Autodesk Inventor part; units mm, degrees
ref_plane "YZ Plane" through (0, 0, 0) normal (1, 0, 0) x (0, 1, 0)
ref_plane "XZ Plane" through (0, 0, 0) normal (0, 1, 0) x (-1, 0, 0)
ref_plane "XY Plane" through (0, 0, 0) normal (0, 0, 1) x (1, 0, 0)
sketch "Sketch1" plane through (0, 0, 0) normal (0, 1, 0) x (-1, 0, 0)
  line L0 (46.6228, 34.6302) -> (-74.0272, 34.6302)
  line L1 (-74.0272, 34.6302) -> (-74.0272, -28.8698)
  line L2 (-74.0272, -28.8698) -> (46.6228, -28.8698)
  line L3 (46.6228, -28.8698) -> (46.6228, 34.6302)
  point P0 (0, 0)
  dimension "d0" = 120.65
  dimension "d1" = 63.5
extrude "Extrusion1" add sketch "Sketch1" along normal blind 12.7
sketch "Sketch2" plane through (0, 12.7, 0) normal (0, 1, 0) x (1, 0, 0)
  line L0 (-46.6228, -34.6302) -> (74.0272, -34.6302)
  line L1 (-46.6228, 28.8698) -> (-46.6228, -34.6302)
  point P0 (0, 0)
  point P1 (4.1772, -18.7552)
  point P2 (54.9772, -18.7552)
  dimension "d4" = 0
  dimension "d5" = 15.875
  dimension "d6" = 50.8
  dimension "d7" = 50.8
hole "Hole1" at (4.1772, 12.7, 18.7552) at (54.9772, 12.7, 18.7552) direction (0, -1, 0) diameter 4.826 depth 25.4 tip angle 118 countersink diameter 9.525 countersink angle 82
sketch "Sketch3" plane through (0, 0, 0) normal (0, -1, 0) x (1, 0, 0)
  line L0 (-16.8428, 29.5502) -> (-28.8428, 29.5502)
  line L1 (-28.8428, 29.5502) -> (-28.8428, 23.5502)
  line L2 (-28.8428, 23.5502) -> (-16.8428, 23.5502)
  line L3 (-16.8428, 23.5502) -> (-16.8428, 29.5502)
  line L4 (-46.6228, 34.6302) -> (74.0272, 34.6302)
  line L5 (-46.6228, -28.8698) -> (-46.6228, 34.6302)
  point P0 (0, 0)
  dimension "d15" = 6
  dimension "d16" = 12
  dimension "d17" = 5.08
  dimension "d18" = 17.78
extrude "Extrusion2" cut sketch "Sketch3" against normal blind 1.27
sketch "Sketch4" plane through (0, 0, 0) normal (0, -1, 0) x (1, 0, 0)
  line L0 (74.0272, -28.8698) -> (-46.6228, -28.8698)
  line L1 (-28.8428, 23.5502) -> (-28.8428, 29.5502)
  line L2 (-46.6228, -28.8698) -> (-46.6228, 34.6302)
  point P0 (0, 0)
  point P1 (-32.8428, -16.6898)
  point P2 (-32.8428, -23.7898)
  point P3 (-11.9428, -23.7898)
  point P4 (-11.9428, -16.6898)
  dimension "d21" = 0
  dimension "d22" = 0
  dimension "d23" = 0
  dimension "d24" = 0
  dimension "d25" = 5.08
  dimension "d26" = 7.1
  dimension "d27" = 20.9
  dimension "d35" = 4
  dimension "d92" = 13.78
hole "Hole2" at (-32.8428, 0, -16.6898) at (-32.8428, 0, -23.7898) at (-11.9428, 0, -23.7898) at (-11.9428, 0, -16.6898) direction (0, 1, 0) diameter 2.8 depth 25.4 tip angle 118
sketch "Sketch6" plane through (0, 0, 0) normal (0, -1, 0) x (1, 0, 0)
  line L0 (-46.6228, 34.6302) -> (74.0272, 34.6302)
  line L1 (-46.6228, -28.8698) -> (-46.6228, 34.6302)
  line L2 (74.0272, -28.8698) -> (-46.6228, -28.8698)
  point P0 (0, 0)
  point P1 (69.7092, -24.6788)
  point P2 (-42.0508, -24.6788)
  point P3 (-42.0508, 30.4392)
  point P4 (69.7092, 30.4392)
  dimension "d43" = 0
  dimension "d44" = 0
  dimension "d46" = 111.76
  dimension "d47" = 0
  dimension "d48" = 0
  dimension "d50" = 4.191
  dimension "d51" = 4.572
  dimension "d91" = 4.191
hole "Hole4" at (69.7092, 0, -24.6788) at (-42.0508, 0, -24.6788) at (-42.0508, 0, 30.4392) at (69.7092, 0, 30.4392) direction (0, 1, 0) diameter 4.8 depth 25.4 tip angle 118
sketch "Sketch10" plane through (0, 12.7, 0) normal (0, 1, 0) x (1, 0, 0)
  circle A0 centre (54.9772, -18.7552) radius 2.413
  circle A1 centre (4.1772, -18.7552) radius 2.413
  line L0 (74.0272, 28.8698) -> (-46.6228, 28.8698)
  point P0 (0, 0)
  point P1 (4.1772, 12.9948)
  point P2 (54.9772, 12.9948)
  point P3 (66.6772, 28.8698)
  point P4 (-45.6228, 28.8698)
  dimension "d80" = 0
  dimension "d81" = 0
  dimension "d82" = 0
  dimension "d83" = 15.875
hole "Hole7" at (4.1772, 12.7, -12.9948) at (54.9772, 12.7, -12.9948) direction (0, -1, 0) diameter 4.826 end through all countersink diameter 9.525 countersink angle 82
sketch "Sketch11" plane through (0, 0, 0) normal (0, -1, 0) x (1, 0, 0)
  line L0 (-28.8428, 6.3402) -> (-16.8428, 6.3402)
  line L1 (-16.8428, 6.3402) -> (-16.8428, 0.3402)
  line L2 (-16.8428, 0.3402) -> (-28.8428, 0.3402)
  line L3 (-28.8428, 0.3402) -> (-28.8428, 6.3402)
  line L4 (-28.8428, -17.7898) -> (-16.8428, -17.7898)
  line L5 (-16.8428, -17.7898) -> (-16.8428, -23.7898)
  line L6 (-16.8428, -23.7898) -> (-28.8428, -23.7898)
  line L7 (-28.8428, -23.7898) -> (-28.8428, -17.7898)
  line L8 (-28.8428, 23.5502) -> (-28.8428, 29.5502)
  line L9 (-16.8428, 29.5502) -> (-16.8428, 23.5502)
  line L10 (74.0272, -28.8698) -> (-46.6228, -28.8698)
  point P0 (0, 0)
  dimension "d93" = 0
  dimension "d94" = 0
  dimension "d95" = 0
  dimension "d96" = 0
  dimension "d97" = 6
  dimension "d98" = 6
  dimension "d99" = 5.08
  dimension "d100" = 29.21
extrude "Extrusion4" cut sketch "Sketch11" against normal blind 1.27
sketch "Sketch12" plane through (0, 0, 0) normal (0, -1, 0) x (1, 0, 0)
  circle A0 centre (-42.0508, 30.4392) radius 2.4
  circle A1 centre (69.7092, 30.4392) radius 2.4
  circle A2 centre (69.7092, -24.6788) radius 2.4
  circle A3 centre (-42.0508, -24.6788) radius 2.4
  point P0 (0, 0)
hole "Hole8" at (-42.0508, 0, 30.4392) at (69.7092, 0, 30.4392) at (69.7092, 0, -24.6788) at (-42.0508, 0, -24.6788) direction (0, 1, 0) diameter 4.826 end through all
sketch "Sketch13" plane through (0, 0, 0) normal (0, -1, 0) x (1, 0, 0)
  circle A0 centre (-32.8428, -16.6898) radius 1.4
  circle A1 centre (-32.8428, -23.7898) radius 1.4
  line L0 (-46.6228, 34.6302) -> (74.0272, 34.6302)
  circle A2 centre (-11.9428, -16.6898) radius 1.4
  point P0 (0, 0)
  point P1 (-32.8428, -0.1798)
  point P2 (-32.8428, 6.9322)
  point P3 (-32.8428, 22.9462)
  point P4 (-32.8428, 30.0582)
  point P5 (-39.7887, 34.6302)
  point P6 (67.4471, 34.6302)
  point P7 (-11.9428, -0.1798)
  point P8 (-11.9428, 6.9322)
  point P9 (-11.9428, 22.9462)
  point P10 (-11.9428, 30.0582)
  dimension "d110" = 0
  dimension "d111" = 0
  dimension "d112" = 0
  dimension "d113" = 7.112
  dimension "d114" = 7.112
  dimension "d115" = 16.51
  dimension "d116" = 4.572
  dimension "d117" = 0
  dimension "d118" = 0
  dimension "d119" = 0
  dimension "d120" = 0
  dimension "d121" = 0
  dimension "d122" = 0
  dimension "d123" = 0
  dimension "d124" = 0
hole "Hole9" at (-32.8428, 0, -0.1798) at (-32.8428, 0, 6.9322) at (-32.8428, 0, 22.9462) at (-32.8428, 0, 30.0582) at (-11.9428, 0, -0.1798) at (-11.9428, 0, 6.9322) at (-11.9428, 0, 22.9462) at (-11.9428, 0, 30.0582) direction (0, 1, 0) diameter 2.8 end through all
sketch "Sketch15" plane through (0, 12.7, 0) normal (0, 1, 0) x (1, 0, 0)
  circle A0 centre (4.1772, 12.9948) radius 2.413
  circle A1 centre (54.9772, 12.9948) radius 2.413
  circle A2 centre (4.1772, -18.7552) radius 2.413
  circle A3 centre (54.9772, -18.7552) radius 2.413
  circle A4 centre (4.1772, 12.9948) radius 3.3734
  circle A5 centre (4.1772, -18.7552) radius 3.3734
  circle A6 centre (54.9772, -18.7552) radius 3.3734
  circle A7 centre (54.9772, 12.9948) radius 3.3734
  point P0 (0, 0)
  dimension "d138" = 6.7469
  dimension "d139" = 6.7469
  dimension "d140" = 6.7469
  dimension "d141" = 6.7469
extrude "Extrusion6" cut sketch "Sketch15" against normal blind 8.89
equation "\"d1\" = 2 * TalonSRXWidth"
equation "\"d15\" = CanConPinWidth"
equation "\"d16\" = CanConPinLength"
equation "\"d28\" = CanConHoleDiam"
equation "\"d52\" = LegoMainHole"
equation "\"d125\" = CanConHoleDiam"
equation "\"LegoMainHole\" = 4.8"
equation "\"TalonSRXWidth\" = 31.75"
equation "\"TalonSRXFromSide\" = 15.875"
equation "\"TalonSRXBetweenHoles\" = 50.8"
equation "\"CanConPinWidth\" = 6"
equation "\"CanConPinLength\" = 12"
equation "\"CanConBetweenSideHoles\" = 20.9"
equation "\"CanConBetweenTopHoles\" = 7.1"
equation "\"CanConHoleDiam\" = 2.8"
equation "\"CanConHoleFromTopPin\" = 4"
properties part number "TalonSRXPlateTwo"
Could you check a few things on this model? Use its own coordinates, in mm. A direction names the side the tool comes from. Round coordinates to 2 decimals unless told otherwise and drop trailing zeros. Write each loop counter-clockwise with the first axis right and the second up, starting at its lowest first coordinate (ties: lowest second). Pieces come first, ordered by that corner, then holes. Notation, with made-up numbers: (7, 64.25) -> (20, 64.25) arc R14 cw to (20, 79.25) -> close; hole circle Ø4 at (68.5, -29). An arc over 180 degrees is marked (long way). Use a Markdown table: item, result.
1. If we section it at A-A (y = 6): State how many separate pieces and enclosed holes the cut face has, then the cut area to 3 significant figures.
Answer key:
| item | result |
|---|---|
| separate pieces | 1 |
| enclosed holes | 20 |
| area | 7,370 mm^2 |
2. We'd pull the mould along X, two halves only. Please class faces 3 (the face through (-46.623, 6, 2)), 4 (the face through (74.027, 6, 3)), 5 (the face through (-11.091, 6.439, 24.057)), 6 (the face through (72.065, 6.439, -24.156)): +X half, -X half, draft (parallel to the pull), parting line (faces both ways), or undercut.
Answer key:
| item | result |
|---|---|
| face 3 | -X half |
| face 4 | +X half |
| face 5 | undercut |
| face 6 | undercut |
3. For pin 1 Ø3 at (x, z) = (52, -14.5) entering from +Y; pin 2 Ø5.5 at (x, z) = (54.98, 18.76) entering from +Y; pin 3 Ø2 at (x, z) = (-32.84, 6.93) entering from -Y; pin 4 Ø5.5 at (x, z) = (56.5, 18) entering from +Y, each with a flat end and sliding along its axis, tell me the tip position at first contact or that it passes through.
Answer key:
| item | result |
|---|---|
| pin 1 | stops at y = 12.7 |
| pin 2 | stops at y = 3.81 |
| pin 3 | passes through |
| pin 4 | stops at y = 12.34 |
4. Please list where these lines run through material, in increasing order: probe 1 along X at (y, z) = (10, -16.5); probe 2 along Z at (x, y) = (4, 3.75); probe 3 along X at (y, z) = (1, 5).
Answer key:
| item | result |
|---|---|
| probe 1 | x = -46.62 to -34.23, -31.46 to -13.33, -10.56 to 74.03 |
| probe 2 | z = -28.87 to -15.4, -10.59 to 16.35, 21.16 to 34.63 |
| probe 3 | x = -46.62 to -28.84, -16.84 to 74.03 |
5. Which directions (+Z, -Z, +X, -X, +Y, -Y) give clear straight access to the entire face, cutting with the end or side of a thin tool? Please do faces 1 (the face through (-39.695, 6.439, -24.156)), 2 (the face through (54, 3.81, 16)).
Answer key:
| item | result |
|---|---|
| face 1 | +Y, -Y |
| face 2 | +Y |
6. If we section it at B-B (x = -19): List the corners of the cut face in (y, z) for me, then the cut area to 3 significant figures.
Answer key:
| item | result |
|---|---|
| outline | (0, -28.87) -> (12.7, -28.87) -> (12.7, 34.63) -> (0, 34.63) -> (0, 29.55) -> (1.27, 29.55) -> (1.27, 23.55) -> (0, 23.55) -> (0, 6.34) -> (1.27, 6.34) -> (1.27, 0.34) -> (0, 0.34) -> (0, -17.79) -> (1.27, -17.79) -> (1.27, -23.79) -> (0, -23.79) -> close |
| area | 784 mm^2 |
